Could you check a few things on this model? Use its own coordinates, in mm. A direction names the side the tool comes from. Coordinates: 2 decimals unless noted, no trailing zeros. Write each loop counter-clockwise with the first axis right and the second up, starting at its lowest first coordinate (ties: lowest second). Pieces come first, ordered by that corner, then holes.
```python
from build123d import *

# Parameters (mm, degrees)
F0_W     = 57.15
F0_H     = 101.6
F1_DEPTH = 3.175
F2_R     = 0.8255
F3_DEPTH = 3.302
F4_W     = 6.35
F4_H     = 6.35
F5_DEPTH = 3.175


with BuildPart() as f1:
    # F0 (on Top) → F1 (new body)
    with BuildSketch(Plane.XY):
        Rectangle(F0_W, F0_H)
    extrude(amount=F1_DEPTH)

    # F2 (on face) → F3 (cut)
    with BuildSketch(Plane(origin=(-28.575, 0, 0), x_dir=(0, -1, 0), z_dir=(-1, 0, 0))):
        with Locations((0, 1.5875)):
            Circle(F2_R)
        with Locations((25.4, 1.5875)):
            Circle(F2_R)
        with Locations((-25.4, 1.5875)):
            Circle(F2_R)
    extrude(amount=-F3_DEPTH, mode=Mode.SUBTRACT)

    # F4 (on face) → F5 (join)
    with BuildSketch(Plane(origin=(0, 0, 0), x_dir=(1, 0, 0), z_dir=(0, 0, -1))):
        with Locations((-25.4, 32.639)):
            Rectangle(F4_W, F4_H)
        with Locations((-25.4, -32.639)):
            Rectangle(F4_W, F4_H)
        with Locations((16.764, -32.639)):
            Rectangle(F4_W, F4_H)
        with Locations((16.764, 32.639)):
            Rectangle(F4_W, F4_H)
    extrude(amount=F5_DEPTH)


solid = f1.part
```
1. I want a section at C-C on y = 15. Please give me the cut outline in (x, z) (3 decimals), plus the area to 3 significant figures.
Verdict:
outline: (-28.575, 0) - (28.575, 0) - (28.575, 3.175) - (-28.575, 3.175) - close
area: 181 mm2
2. On a 3-axis mill with a long thin cutter (end or side, diameter ignored), from which of +Z, -Z, +X, -X, +Y, -Y can I reach the whole of each face in a straight line? I mean faces 1 (the face through (13.589, -33, -2)), 2 (the face through (17, -35.814, -2)), 3 (the face through (19.939, -33, -2)). Say none if no direction works.
Verdict:
face 1: -Z, +Y, -Y
face 2: -Z, +X, -X, -Y
face 3: -Z, +X, +Y, -Y
3. I want a section at B-B on x = 25.5. Please give me the cut outline in (y, z) (3 decimals).
Verdict:
outline: (-50.8, 0) - (50.8, 0) - (50.8, 3.175) - (-50.8, 3.175) - close
4. For pin 1 (1.3 mm diameter, centred on y = 0, z = 1.59, fed in from -X); pin 2 (2.5 mm diameter, centred on y = 33.5, z = -1.5, fed in from +X); pin 3 (1 mm diameter, centred on x = -24.5, z = -1, fed in from -Y); pin 4 (2 mm diameter, centred on y = -3, z = -0.5, fed in from -X) (3 decimals), each with a flat end and sliding along its axis, tell me the tip position at first contact or that it passes through.
Verdict:
pin 1: stops at x = -25.27
pin 2: stops at x = 19.94
pin 3: stops at y = -35.81
pin 4: stops at x = -28.575
5. If we mould it in two halves opening along Y, with no side actions, what happens to faces 4 (the face through (17, 35.814, -2)), 5 (the face through (-25, -29.464, -2)), 6 (the face through (17, 29.464, -2)), 7 (the face through (-28.575, -1, 1))? For each: pulls with the +Y half, pulls with the -Y half, needs draft (parallel to the pull), parting line crosses it, or undercut.
Verdict:
face 4: pulls with the +Y half
face 5: undercut
face 6: undercut
face 7: needs draft
6. I want a section at A-A on y = -32. Please give me the cut outline in (x, z) (3 decimals), plus the area to 3 significant figures.
Verdict:
outline: (-28.575, -3.175) - (-22.225, -3.175) - (-22.225, 0) - (13.589, 0) - (13.589, -3.175) - (19.939, -3.175) - (19.939, 0) - (28.575, 0) - (28.575, 3.175) - (-28.575, 3.175) - close
area: 222 mm2
7. Please list where these lines run through material, in increasing order: line 1 along Z through (x, y) = (-26.4, 0) (3 decimals); line 2 along Y through (x, z) = (-25.5, 1); line 3 along X through (y, z) = (30.5, -0.75) (3 decimals).
Verdict:
line 1: z = 0 to 0.762, 2.413 to 3.175
line 2: y = -50.8 to -25.98, -24.82 to -0.58, 0.58 to 24.82, 25.98 to 50.8
line 3: x = -28.575 to -22.225, 13.589 to 19.939
